CAD build for the part. Positions are in the model's coordinates, mm. A direction names the side the tool comes from. Round coordinates to 2 decimals unless told otherwise and drop trailing zeros. Order: outer loops, then holes, each group sorted by start corner. A loop starts at its lowest first (then second) coordinate and runs counter-clockwise, first axis right, second up. Notation, with made-up numbers: (34, 26.25) - (50, 26.25) arc R14 cw to (50, 33.25) - close; hole circle Ø5 at (-24.75, 70). An arc over 180 degrees is marked (long way). Use one line per item in the form item = value. Start each with the question number.
from build123d import *

# Parameters (mm, degrees)
F0_W     = 165.1
F0_H     = 114.3
F1_DEPTH = 12.7
F2_R     = 38.1
F2_R_2   = 31.75
F3_DEPTH = 50.8
F4_R     = 5.49275
F4_R_2   = 7.14375
F5_DEPTH = 25.4
F7_DEPTH = 76.2


with BuildPart() as f1:
    # F0 (on Top) → F1 (new body)
    with BuildSketch(Plane.XY):
        with Locations((82.55, 57.15)):
            Rectangle(F0_W, F0_H)
    extrude(amount=F1_DEPTH)

    # F2 (on face) → F3 (join)
    with BuildSketch(Plane.XY.offset(12.7)):
        with Locations((82.55, 57.15)):
            Circle(F2_R)
        with Locations((82.55, 57.15)):
            Circle(F2_R_2, mode=Mode.SUBTRACT)
    extrude(amount=F3_DEPTH)

    # F4 (on face) → F5 (cut)
    with BuildSketch(Plane.XY.offset(12.7)):
        with Locations((152.4, 57.15)):
            Circle(F4_R)
        with Locations((12.7, 57.15)):
            Circle(F4_R)
        with Locations((82.55, 57.15)):
            Circle(F4_R_2)
    extrude(amount=-F5_DEPTH, mode=Mode.SUBTRACT)

    # F6 (on Front) → F7 (cut)
    with BuildSketch(Plane.XZ):
        with BuildLine():
            ThreePointArc((79.375, 19.05), (82.55, 15.875), (85.725, 19.05))
            ThreePointArc((85.725, 19.05), (82.55, 22.225), (79.375, 19.05))
        make_face()
    extrude(amount=-F7_DEPTH, mode=Mode.SUBTRACT)


solid = f1.part
(1) Slice it at A-A (x = 152.4). Give the cut face in (y, z).
(2) Flat gauge pins, fed straight in: P1, Ø10, axis at x = 82.55, z = 19.05, coming from the -Y side; P2, Ø2, axis at x = 102.5, y = 36, coming from the +Z side; P3, Ø4, axis at y = 57.5, z = 19, coming from the +X side; P4, Ø1, axis at x = 142, y = 13.5, coming from the -Z side. Where does each tip first touch, or does it go through?
(3) Mould opens along Y. For faces 1 (the flat face through (45, 71, 12.7)), 2 (the cylindrical face through (157.474, 55.046, 6.439)), 3 (the flat face through (81, 114.3, 6)), 4 (the cylindrical face through (74.291, 19.956, 37.744)) say: pulls with the +Y half, pulls with the -Y half, needs draft (parallel to the pull), parting line crosses it, or undercut.
(4) Which spindle directions (+Z, -Z, +X, -X, +Y, -Y) get a long thin tool onto all of the face, cutting with end or side? Do faces 5 (the flat face through (75, 58, 12.7)), 6 (the cylindrical face through (85.58, 22.26, 20)), 7 (the flat face through (81, 71, 0)). Say none if no direction does.
(5) Slice it at C-C (z = 8). Give the cut face in (x, y).
(6) Wall check: line 1 (X direction, y = 57, z = 4); line 2 (Y direction, x = 152, z = 3); line 3 (Y direction, x = 82.55, z = 4.5). Give the ranges that are in metal, low to high. Write a range as [from, to].
(7) Slice it at D-D (x = 82.55). Give the cut face in (y, z) (3 decimals), and give its area (4 significant figures).
(8) Slice it at B-B (y = 57.15). Give the cut face in (x, z), and give its area (3 significant figures).
Results list:
q1.outline = (0, 0) - (51.66, 0) - (51.66, 12.7) - (0, 12.7) - close; (62.64, 0) - (114.3, 0) - (114.3, 12.7) - (62.64, 12.7) - close
q2.P1 = 19.05
q2.P2 = 12.7
q2.P3 = 120.65
q2.P4 = 0
q3.face_1 = needs draft
q3.face_2 = undercut
q3.face_3 = pulls with the +Y half
q3.face_4 = parting line crosses it
q4.face_5 = +Z
q4.face_6 = -Y
q4.face_7 = -Z, +X, -X, +Y, -Y
q5.outline = (0, 0) - (165.1, 0) - (165.1, 114.3) - (0, 114.3) - close; hole circle Ø10.99 at (12.7, 57.15); hole circle Ø14.29 at (82.55, 57.15); hole circle Ø10.99 at (152.4, 57.15)
q6.line_1 = [0, 7.21], [18.19, 75.41], [89.69, 146.91], [157.89, 165.1]
q6.line_2 = [0, 51.67], [62.63, 114.3]
q6.line_3 = [0, 50.01], [64.29, 114.3]
q7.outline = (0, 0) - (50.006, 0) - (50.006, 12.7) - (25.4, 12.7) - (25.4, 15.875) - (19.05, 15.875) - (19.05, 12.7) - (0, 12.7) - close; (19.05, 22.225) - (25.4, 22.225) - (25.4, 63.5) - (19.05, 63.5) - close; (64.294, 0) - (114.3, 0) - (114.3, 12.7) - (95.25, 12.7) - (95.25, 63.5) - (88.9, 63.5) - (88.9, 12.7) - (64.294, 12.7) - close
q7.area = 1,875 mm²
q8.outline = (0, 0) - (7.21, 0) - (7.21, 12.7) - (0, 12.7) - close; (18.19, 0) - (75.41, 0) - (75.41, 12.7) - (50.8, 12.7) - (50.8, 63.5) - (44.45, 63.5) - (44.45, 12.7) - (18.19, 12.7) - close; (89.69, 0) - (146.91, 0) - (146.91, 12.7) - (120.65, 12.7) - (120.65, 63.5) - (114.3, 63.5) - (114.3, 12.7) - (89.69, 12.7) - close; (157.89, 0) - (165.1, 0) - (165.1, 12.7) - (157.89, 12.7) - close
q8.area = 2,280 mm²
